Here's how the part is built. I have some questions about the finished solid (model axes, mm). A direction names the side the tool comes from. Coordinates: 2 decimals unless noted, no trailing zeros. Order: outer loops, then holes, each group sorted by start corner. A loop starts at its lowest first (then second) coordinate and runs counter-clockwise, first axis right, second up.
Autodesk Inventor part; units mm, degrees
ref_plane "YZ Plane" through (0, 0, 0) normal (1, 0, 0) x (0, 1, 0)
ref_plane "XZ Plane" through (0, 0, 0) normal (0, 1, 0) x (-1, 0, 0)
ref_plane "XY Plane" through (0, 0, 0) normal (0, 0, 1) x (1, 0, 0)
sketch "Sketch1" plane through (0, 0, 0) normal (0, 0, 1) x (1, 0, 0)
  circle A0 centre (27.386, 18.5258) radius 21
  circle A1 centre (27.386, 18.5258) radius 17
  dimension "d0" = 42
  dimension "d1" = 34
extrude "Outer" add sketch "Sketch1" along normal blind 1
sketch "Sketch2" plane through (27.386, 18.5258, 1) normal (0, 0, 1) x (1, 0, 0)
  circle A0 centre (0, 0) radius 17.5
  dimension "d4" = 35
extrude "Breath_ext_outer" add sketch "Sketch2" against normal blind 10
sketch "Sketch3" plane through (27.386, 18.5258, 1) normal (0, 0, 1) x (1, 0, 0)
  circle A0 centre (0, 0) radius 17
  dimension "d7" = 34
extrude "Breath_ext_inner" cut sketch "Sketch3" against normal blind 9
sketch "Sketch4" plane through (27.386, 18.5258, -9) normal (0, 0, -1) x (-1, 0, 0)
  arc A0 (-10.3804, 2.7946) -> (-10.3234, -2.9983) centre (0, 0) ccw
  arc A1 (-13.233, 4.5704) -> (-13.2519, -4.5152) centre (0, 0) ccw
  line L0 (-10.3234, -2.9983) -> (-13.2519, -4.5152)
  line L1 (-10.3804, 2.7946) -> (-13.233, 4.5704)
  arc A2 (-2.7701, 10.387) -> (-7.7583, 7.4412) centre (0, 0) ccw
  arc A3 (-2.6584, 13.7453) -> (-10.5362, 9.2189) centre (0, 0) ccw
  line L2 (-7.7583, 7.4412) -> (-10.5362, 9.2189)
  line L3 (-2.7701, 10.387) -> (-2.6584, 13.7453)
  arc A4 (7.6104, 7.5924) -> (2.5651, 10.4395) centre (0, 0) ccw
  arc A5 (10.5746, 9.1749) -> (2.7157, 13.7341) centre (0, 0) ccw
  line L4 (2.5651, 10.4395) -> (2.7157, 13.7341)
  line L5 (7.6104, 7.5924) -> (10.5746, 9.1749)
  arc A6 (10.3804, -2.7946) -> (10.3234, 2.9983) centre (0, 0) ccw
  arc A7 (13.233, -4.5704) -> (13.2519, 4.5152) centre (0, 0) ccw
  line L6 (10.3234, 2.9983) -> (13.2519, 4.5152)
  line L7 (10.3804, -2.7946) -> (13.233, -4.5704)
  arc A8 (2.7701, -10.387) -> (7.7583, -7.4412) centre (0, 0) ccw
  arc A9 (2.6584, -13.7453) -> (10.5362, -9.2189) centre (0, 0) ccw
  line L8 (7.7583, -7.4412) -> (10.5362, -9.2189)
  line L9 (2.7701, -10.387) -> (2.6584, -13.7453)
  arc A10 (-7.6104, -7.5924) -> (-2.5651, -10.4395) centre (0, 0) ccw
  arc A11 (-10.5746, -9.1749) -> (-2.7157, -13.7341) centre (0, 0) ccw
  line L10 (-2.5651, -10.4395) -> (-2.7157, -13.7341)
  line L11 (-7.6104, -7.5924) -> (-10.5746, -9.1749)
  dimension "d14" = 360
extrude "Breath_Holes" cut sketch "Sketch4" against normal blind 2
sketch "Sketch5" plane through (27.386, 18.5258, -8) normal (0, 0, 1) x (1, 0, 0)
  circle A0 centre (0, 0) radius 3
  dimension "d18" = 6
extrude "Hole_holder" add sketch "Sketch5" along normal blind 8
sketch "Sketch6" plane through (27.386, 18.5258, 0) normal (0, 0, 1) x (1, 0, 0)
  point P0 (0, 0.0702)
hole "Hole1" at (27.386, 18.596, 0) direction (0, 0, -1) diameter 2.1 depth 7 tip angle 118 counterbore diameter 3 counterbore depth 1
properties part number "mask_breath_top"
Q1. I need wall thicknesses on L1, parallel to Z at x = 16, y = 30.5; L2, parallel to X at y = 29, z = -8.5; L3, parallel to X at y = 11, z = -2.25. Which ranges of each line are inside material? Lowest first, please.
Q2. For faces 1 (the flat face through (30.025, 6.462, -8.507)), 2 (the cylindrical face through (24.39, 18.39, -4.06)), which set-ups out of +Z, -Z, +X, -X, +Y, -Y let a thin tool reach every point of the face, with its end or its side?
Q3. If we section it at C-C on z = -0.5: Write out the boundary of the cut face in (x, y).
Q4. If we section it at D-D on y = 25: Write out the boundary of the cut face in (x, z), then the cut area to 3 significant figures.
Q5. Will these pins go through, and if not, where does the flat tip stop? pin 1 (1.5 mm diameter, centred on x = 31, z = -1.5, fed in from -Y); pin 2 (4 mm diameter, centred on x = 27.386, y = 18.596, fed in from +Z); pin 3 (1 mm diameter, centred on x = 31.5, z = -3, fed in from +Y).
Q6. If we section it at B-B on x = 18.5: Write out the boundary of the cut face in (y, z).
Q7. If we section it at A-A on y = 7: Write out the boundary of the cut face in (x, z).
Q8. We'd pull the mould along Y, two halves only. Please class faces 3 (the flat face through (35, 3, 1)), 4 (the cylindrical face through (47.416, 12.218, 0.493)), 5 (the cylindrical face through (16.636, 18.591, -8.507)): pulls with the +Y half, pulls with the -Y half, needs draft (parallel to the pull), parting line crosses it, or undercut.
Reply:
1. L1: z = -9 to -8
1. L2: x = 13.37 to 18.1, 24.82 to 30.15, 36.68 to 41.41
1. L3: x = 11.59 to 12.14, 42.63 to 43.19
2. face 1: +Z, -Z
2. face 2: +Z
3. outline: circle Ø35 at (27.39, 18.53); circle Ø6 at (27.39, 18.53); hole circle Ø34 at (27.39, 18.53); hole circle Ø3 at (27.39, 18.6)
4. outline: (7.41, 0) - (11.13, 0) - (11.13, -9) - (43.64, -9) - (43.64, 0) - (47.36, 0) - (47.36, 1) - (43.1, 1) - (43.1, -8) - (11.67, -8) - (11.67, 1) - (7.41, 1) - close
4. area: 49.7 mm2
5. pin 1: stops at y = 1.26
5. pin 2: stops at z = 0
5. pin 3: stops at y = 35.65
6. outline: (-0.5, 0) - (3.45, 0) - (3.45, -9) - (7.71, -9) - (7.71, -8) - (4.03, -8) - (4.03, 1) - (-0.5, 1) - close; (10.36, -9) - (26.8, -9) - (26.8, -8) - (10.36, -8) - close; (29.34, -9) - (33.6, -9) - (33.6, 0) - (37.55, 0) - (37.55, 1) - (33.02, 1) - (33.02, -8) - (29.34, -8) - close
7. outline: (9.83, 0) - (14.22, 0) - (14.22, -9) - (19.44, -9) - (19.44, -8) - (14.89, -8) - (14.89, 1) - (9.83, 1) - close; (24.65, -9) - (30, -9) - (30, -8) - (24.65, -8) - close; (35.33, -9) - (40.55, -9) - (40.55, 0) - (44.94, 0) - (44.94, 1) - (39.88, 1) - (39.88, -8) - (35.33, -8) - close
8. face 3: needs draft
8. face 4: parting line crosses it
8. face 5: undercut
